Autodesk Inventor part; units mm, degrees
ref_plane "YZ Plane" through (0, 0, 0) normal (1, 0, 0) x (0, 1, 0)
ref_plane "XZ Plane" through (0, 0, 0) normal (0, 1, 0) x (-1, 0, 0)
ref_plane "XY Plane" through (0, 0, 0) normal (0, 0, 1) x (1, 0, 0)
sketch "Sketch1" plane through (0, 0, 0) normal (0, 1, 0) x (-1, 0, 0)
  line L0 (36.5552, 136.6167) -> (36.5552, 130.2667)
  line L1 (21.3152, 130.2667) -> (21.3152, 136.6167)
  line L2 (58.1452, 96.9292) -> (64.4952, 96.9292)
  line L3 (64.4952, 77.8792) -> (58.1452, 77.8792)
  line L4 (58.1452, 52.4792) -> (64.4952, 52.4792)
  line L5 (64.4952, 33.4292) -> (58.1452, 33.4292)
  line L6 (58.1452, 8.0292) -> (64.4952, 8.0292)
  line L7 (64.4952, -1.4958) -> (-62.2762, -1.4958) construction
  line L8 (-7.1455, 136.6167) -> (-7.1455, -139.6083) construction
  line L9 (58.1452, 96.9292) -> (58.1452, 77.8792)
  line L10 (58.1452, 33.4292) -> (58.1452, 52.4792)
  line L11 (36.5552, 130.2667) -> (21.3152, 130.2667)
  line L12 (-50.8462, 136.6167) -> (-50.8462, 130.2667)
  line L13 (-20.3662, 136.6167) -> (-20.3662, 130.2667)
  line L14 (-35.6062, 130.2667) -> (-35.6062, 136.6167)
  line L15 (-78.7862, 122.3292) -> (-72.4362, 122.3292)
  line L16 (-72.4362, 96.9292) -> (-78.7862, 96.9292)
  line L17 (-78.7862, 77.8792) -> (-72.4362, 77.8792)
  line L18 (-72.4362, 52.4792) -> (-78.7862, 52.4792)
  line L19 (-78.7862, 33.4292) -> (-72.4362, 33.4292)
  line L20 (-72.4362, 8.0292) -> (-78.7862, 8.0292)
  line L21 (-72.4362, 96.9292) -> (-72.4362, 77.8792)
  line L22 (-72.4362, 33.4292) -> (-72.4362, 52.4792)
  line L23 (-50.8462, 130.2667) -> (-35.6062, 130.2667)
  line L24 (36.5552, -139.6083) -> (36.5552, -133.2583)
  line L25 (6.0752, -139.6083) -> (6.0752, -133.2583)
  line L26 (21.3152, -133.2583) -> (21.3152, -139.6083)
  line L27 (64.4952, -125.3208) -> (58.1452, -125.3208)
  line L28 (58.1452, -99.9208) -> (64.4952, -99.9208)
  line L29 (64.4952, -80.8708) -> (58.1452, -80.8708)
  line L30 (58.1452, -55.4708) -> (64.4952, -55.4708)
  line L31 (64.4952, -36.4208) -> (58.1452, -36.4208)
  line L32 (58.1452, -11.0208) -> (64.4952, -11.0208)
  line L33 (-7.1455, -139.6083) -> (-7.1455, 136.6167) construction
  line L34 (58.1452, -99.9208) -> (58.1452, -80.8708)
  line L35 (58.1452, -36.4208) -> (58.1452, -55.4708)
  line L36 (36.5552, -133.2583) -> (21.3152, -133.2583)
  line L37 (-72.4362, -55.4708) -> (-78.7862, -55.4708)
  line L38 (-78.7862, -80.8708) -> (-72.4362, -80.8708)
  line L39 (-72.4362, -99.9208) -> (-72.4362, -80.8708)
  line L40 (-50.8462, -139.6083) -> (-50.8462, -133.2583)
  line L41 (-20.3662, -139.6083) -> (-20.3662, -133.2583)
  line L42 (-35.6062, -133.2583) -> (-35.6062, -139.6083)
  line L43 (-72.4362, -99.9208) -> (-78.7862, -99.9208)
  line L44 (-78.7862, -125.3208) -> (-72.4362, -125.3208)
  line L45 (-50.8462, -133.2583) -> (-35.6062, -133.2583)
  line L46 (-72.4362, -36.4208) -> (-72.4362, -55.4708)
  line L47 (-78.7862, -36.4208) -> (-72.4362, -36.4208)
  line L48 (-72.4362, -11.0208) -> (-78.7862, -11.0208)
  line L49 (51.7952, 136.6167) -> (36.5552, 136.6167)
  line L50 (-20.3662, 136.6167) -> (-35.6062, 136.6167)
  line L51 (-50.8462, 136.6167) -> (-66.0862, 136.6167)
  line L52 (64.4952, 96.9292) -> (64.4952, 122.3292)
  line L53 (64.4952, 52.4792) -> (64.4952, 77.8792)
  line L54 (58.1452, 8.0292) -> (58.1452, -11.0208)
  line L55 (64.4952, 8.0292) -> (64.4952, 33.4292)
  line L56 (64.4952, -36.4208) -> (64.4952, -11.0208)
  line L57 (64.4952, -80.8708) -> (64.4952, -55.4708)
  line L58 (58.1452, -125.3208) -> (58.1452, -133.2583)
  line L59 (-72.4362, -133.2583) -> (-72.4362, -125.3208)
  line L60 (-72.4362, 8.0292) -> (-72.4362, -11.0208)
  line L61 (-72.4362, 122.3292) -> (-72.4362, 130.2667)
  line L62 (-78.7862, 122.3292) -> (-78.7862, 96.9292)
  line L63 (-78.7862, 77.8792) -> (-78.7862, 52.4792)
  line L64 (-78.7862, 33.4292) -> (-78.7862, 8.0292)
  line L65 (-78.7862, -11.0208) -> (-78.7862, -36.4208)
  line L66 (-78.7862, -55.4708) -> (-78.7862, -80.8708)
  line L67 (-78.7862, -99.9208) -> (-78.7862, -125.3208)
  line L68 (64.4952, -125.3208) -> (64.4952, -99.9208)
  line L69 (-66.0862, -139.6083) -> (-50.8462, -139.6083)
  line L70 (6.0752, -133.2583) -> (-20.3662, -133.2583)
  line L71 (-35.6062, -139.6083) -> (-20.3662, -139.6083)
  line L72 (6.0752, -139.6083) -> (21.3152, -139.6083)
  line L73 (36.5552, -139.6083) -> (51.7952, -139.6083)
  line L74 (58.1452, 130.2667) -> (51.7952, 130.2667)
  line L75 (51.7952, 130.2667) -> (51.7952, 136.6167)
  line L76 (-66.0862, 136.6167) -> (-66.0862, 130.2667)
  line L77 (-66.0862, -139.6083) -> (-66.0862, -133.2583)
  line L78 (51.7952, -139.6083) -> (51.7952, -133.2583)
  line L79 (6.0752, 130.2667) -> (-20.3662, 130.2667)
  line L80 (-66.0862, 130.2667) -> (-72.4362, 130.2667)
  line L81 (6.0752, 130.2667) -> (6.0752, 136.6167)
  line L82 (21.3152, 136.6167) -> (6.0752, 136.6167)
  line L83 (58.1452, 122.3292) -> (58.1452, 130.2667)
  line L84 (64.4952, 122.3292) -> (58.1452, 122.3292)
  line L85 (51.7952, -133.2583) -> (58.1452, -133.2583)
  line L86 (-66.0862, -133.2583) -> (-72.4362, -133.2583)
  point P0 (0, 0)
  point P1 (58.1452, 136.6167)
  dimension "d4" = 15.24
  dimension "d7" = 9.525
  dimension "d8" = 19.05
  dimension "d9" = 19.05
  dimension "d10" = 25.4
  dimension "d12" = 25.4
  dimension "d18" = 15.24
  dimension "d25" = 143.2814
  dimension "d27" = 6.35
  dimension "d28" = 15.24
  dimension "d29" = 6.35
  dimension "d30" = 15.24
extrude "Extrusion2" add sketch "Sketch1" along normal blind 6.35
equation "\"d4\" = d3"
equation "\"d8\" = 2 * d7"
equation "\"d9\" = d8"
equation "\"d10\" = d12"
equation "\"d12\" = d11"
equation "\"d30\" = d18"
properties part number "Bottom" material "UHMW, White"
Design review of the part built by this model. Coordinates are the model's own, in mm. A direction names the side the tool comes from. Round coordinates to 2 decimals unless told otherwise and drop trailing zeros. Order: outer loops, then holes, each group sorted by start corner. A loop starts at its lowest first (then second) coordinate and runs counter-clockwise, first axis right, second up. Notation, with made-up numbers: M 67,75 L 105,75 A23 cw 105,83 Z; hole C 71.25,9.25 d9. An arc over 180 degrees is marked long. Answer as CSV lines item,"result". Start each with the question number.
1) Add section B-B (x = -27). Give the boundary of the cut face in (y, z).
2) Tool access review of faces 4 (the face through (35.606, 3, -136)), 5 (the face through (69, 3, -133.258)), 6 (the face through (-58.145, 3, 126)), 7 (the face through (76, 3, 33.429)), 8 (the face through (-58.145, 3, 88)): name each direction out of +Z, -Z, +X, -X, +Y, -Y from which nothing blocks a thin tool from reaching the whole face with its end or side.
3) Wall thickness on line 1 along Z through (x, y) = (-31.5, 0.5); line 2 along X through (y, z) = (1.5, -4.5): over which ranges is each line inside the solid? List them lowest first. Write a range as [from, to].
4) Add section A-A (z = 38.5). Give the boundary of the cut face in (x, y), then the cut area to 3 significant figures.
5) The part is to be moulded in two halves that separate along Z. For faces 1 (the face through (-29, 3, 130.267)), 2 (the face through (78.786, 3, -24)), 3 (the face through (-61, 3, 77.879)), say which applies: +Z half, -Z half, draft (parallel to the pull), parting line (faces both ways), or undercut.
6) For pin 1 Ø3 at (x, y) = (77, 2.5) entering from +Z; pin 2 Ø1.9 at (x, y) = (-55, 3) entering from -Z; pin 3 Ø3 at (y, z) = (2.5, -136.5) entering from +X, all flat-tipped, find the tip position at first contact; note any pin that passes through.
Resolved:
1,outline,"M 0,-133.26 L 6.35,-133.26 L 6.35,130.27 L 0,130.27 Z"
2,face 4,"-Z, +Y, -Y"
2,face 5,"-Z, +X, +Y, -Y"
2,face 6,"+Z, -X, +Y, -Y"
2,face 7,"+X, +Y, -Y"
2,face 8,"-X, +Y, -Y"
3,line 1,"[-133.26, 130.27]"
3,line 2,"[-58.15, 72.44]"
4,outline,"M -58.15,0 L 72.44,0 L 72.44,6.35 L -58.15,6.35 Z"
4,area,"829 mm^2"
5,face 1,"+Z half"
5,face 2,"draft"
5,face 3,"undercut"
6,pin 1,"z = 122.33"
6,pin 2,"z = -133.26"
6,pin 3,"x = 66.09"
